```python
from build123d import *

# Parameters (mm, degrees)
F0_W      = 609.6
F0_H      = 431.8
F0_H_2    = 787.4
F1_DEPTH  = 38.1
F2_R      = 5.08
F3_R      = 3.875472852
F4_DEPTH  = 152.4
F5_R      = 3.7758304199
F6_DEPTH  = 152.4
F7_R      = 3.9853573506
F8_DEPTH  = 152.4
F9_R      = 4.2462881123
F10_DEPTH = 152.4
F11_R     = 4.2955728054
F12_DEPTH = 152.4
F13_W     = 600.7608175278
F13_H     = 151.1726528406
F15_DEPTH = 421.64
F14_W     = 862.8795146942
F14_H     = 152.4000018835
F16_DEPTH = 421.64
F17_W     = 11.0756754875
F17_H     = 142.5614315085
F18_DEPTH = 789.94


with BuildPart() as f1:
    # F0 (on Top) → F1 (new body)
    with BuildSketch(Plane.XY):
        with Locations((-304.8, -215.9)):
            Rectangle(F0_W, F0_H)
        with Locations((-304.8, 393.7)):
            Rectangle(F0_W, F0_H_2)
        with Locations((304.8, -215.9)):
            Rectangle(F0_W, F0_H)
    extrude(amount=F1_DEPTH)

    # F2
    f2_edges = [f1.edges().sort_by_distance(p)[0] for p in [
        (0, -431.8, 38.1),
        (609.6, -431.8, 19.05),
        (609.6, -215.9, 38.1),
        (304.8, 0, 38.1),
        (0, 393.7, 38.1),
        (-609.6, 177.8, 38.1),
        (-304.8, 787.4, 38.1),
        (0, 393.7, 0),
        (609.6, 0, 19.05),
        (304.8, 0, 0),
        (0, 0, 19.05),
        (609.6, -215.9, 0),
        (0, 787.4, 19.05),
        (-304.8, 787.4, 0),
        (-609.6, 787.4, 19.05),
        (-609.6, -431.8, 19.05),
        (-609.6, 177.8, 0),
        (0, -431.8, 0),
    ]]
    fillet(f2_edges, radius=F2_R)

    # F3 (on face) → F4 (join)
    with BuildSketch(Plane(origin=(0, 0, 0), x_dir=(1, 0, 0), z_dir=(0, 0, -1))):
        with Locations((-604.52, -782.32)):
            Circle(F3_R)
    extrude(amount=F4_DEPTH)

    # F5 (on face) → F6 (join)
    with BuildSketch(Plane(origin=(0, 0, 0), x_dir=(1, 0, 0), z_dir=(0, 0, -1))):
        with Locations((-604.52, 426.72)):
            Circle(F5_R)
    extrude(amount=F6_DEPTH)

    # F7 (on face) → F8 (join)
    with BuildSketch(Plane(origin=(0, 0, 0), x_dir=(1, 0, 0), z_dir=(0, 0, -1))):
        with Locations((604.52, 426.72)):
            Circle(F7_R)
    extrude(amount=F8_DEPTH)

    # F9 (on face) → F10 (join)
    with BuildSketch(Plane(origin=(0, 0, 0), x_dir=(1, 0, 0), z_dir=(0, 0, -1))):
        with Locations((604.52, 5.08)):
            Circle(F9_R)
    extrude(amount=F10_DEPTH)

    # F11 (on face) → F12 (join)
    with BuildSketch(Plane(origin=(0, 0, 0), x_dir=(1, 0, 0), z_dir=(0, 0, -1))):
        with Locations((-5.08, -782.32)):
            Circle(F11_R)
    extrude(amount=F12_DEPTH)

    # F13 (on Front) → F15 (join)
    with BuildSketch(Plane.XZ):
        with Locations((300.3804087639, -75.5863264203)):
            Rectangle(F13_W, F13_H)
    extrude(amount=F15_DEPTH)

    # F14 (on Front) → F16 (join)
    with BuildSketch(Plane.XZ):
        with Locations((-172.0642447472, -76.2000009418)):
            Rectangle(F14_W, F14_H)
    extrude(amount=F16_DEPTH)

    # F17 (on Front) → F18 (join)
    with BuildSketch(Plane.XZ):
        with Locations((-597.8262126446, -77.9886713717)):
            Rectangle(F17_W, F17_H)
    extrude(amount=-F18_DEPTH)


solid = f1.part
```
Geometry: final body of the model. Coordinates: model frame, mm. A direction names the side the tool comes from. Round coordinates to 2 decimals unless told otherwise and drop trailing zeros. Write each loop counter-clockwise with the first axis right and the second up, starting at its lowest first coordinate (ties: lowest second). Pieces come first, ordered by that corner, then holes. Notation, with made-up numbers: M 40.5,49 L 53.5,49 A27 cw 53.5,72 Z; hole C 40.5,37.25 d3. An arc over 180 degrees is marked long. Answer in a Markdown table with one row per item. Add a question column.
(1) Reachability of faces 1 (the face through (-603.504, -208, -77)), 2 (the face through (301, 0, 19)), 3 (the face through (609.6, -219, 19)) from +Z, -Z, +X, -X, +Y, -Y: full face, straight path, thin tool, end or side. Return the list, or none.
(2) Cut plane D-D, the plane x = 240. Return the cut outline in (y, z).
(3) Contact query for flat-ended pins moving along their axis: pin 1 (9 mm diameter, centred on x = -599, y = 377.5, fed in from -Z); pin 2 (1.5 mm diameter, centred on y = 417.5, z = -89, fed in from -X); pin 3 (0.6 mm diameter, centred on y = -300, z = -152, fed in from +X). Output: stop coordinate, or through.
(4) Cut plane C-C, the plane x = 467. Return the cut outline in (y, z), then the cut area to 3 significant figures.
(5) Cut plane A-A, the plane y = 29. Return the cut outline in (x, z).
(6) Ray query, L1, parallel to Y at x = -477, z = -30; L2, parallel to X at y = 325, z = -122.5; L3, parallel to Z at x = 443.5, y = -322. Return the intervals inside material, ascending.
(7) Cut plane B-B, the plane z = -95.5. Return the cut outline in (x, y), then the cut area to 3 significant figures.
Established:
| question | item | result |
|---|---|---|
| 1 | face 1 | -Z, -X |
| 1 | face 2 | +Z, -Z, +X, +Y |
| 1 | face 3 | +Z, -Z, +X, +Y, -Y |
| 2 | outline | M -431.8,5.08 A5.08 ccw -426.72,0 L -421.64,0 L -421.64,-152.4 L 0,-152.4 L 0,0 L -5.08,0 A5.08 ccw 0,5.08 L 0,33.02 A5.08 ccw -5.08,38.1 L -426.72,38.1 A5.08 ccw -431.8,33.02 Z |
| 3 | pin 1 | z = -149.27 |
| 3 | pin 2 | x = -603.36 |
| 3 | pin 3 | x = 259.38 |
| 4 | outline | M -431.8,5.08 A5.08 ccw -426.72,0 L -421.64,0 L -421.64,-151.17 L 0,-151.17 L 0,0 L -5.08,0 A5.08 ccw 0,5.08 L 0,33.02 A5.08 ccw -5.08,38.1 L -426.72,38.1 A5.08 ccw -431.8,33.02 Z |
| 4 | area | 80,200 mm² |
| 5 | outline | M -609.6,5.08 A5.08 ccw -604.52,0 L -5.08,0 A5.08 ccw 0,5.08 L 0,33.02 A5.08 ccw -5.08,38.1 L -604.52,38.1 A5.08 ccw -609.6,33.02 Z; M -603.36,-149.27 L -592.29,-149.27 L -592.29,-6.71 L -603.36,-6.71 Z |
| 6 | L1 | -421.64 to 0 |
| 6 | L2 | -603.36 to -592.29 |
| 6 | L3 | -151.17 to 38.1 |
| 7 | outline | C -604.52,-426.72 d7.55; M -603.5,-421.64 L 600.76,-421.64 L 600.76,-7.05 A4.25 ccw long 600.76,-3.11 L 600.76,0 L -592.29,0 L -592.29,789.94 L -603.36,789.94 L -603.36,786.02 A3.88 ccw long -603.36,778.62 L -603.36,0 L -603.5,0 Z; C -5.08,782.32 d8.59; C 604.52,-426.72 d7.97 |
| 7 | area | 517,000 mm² |
